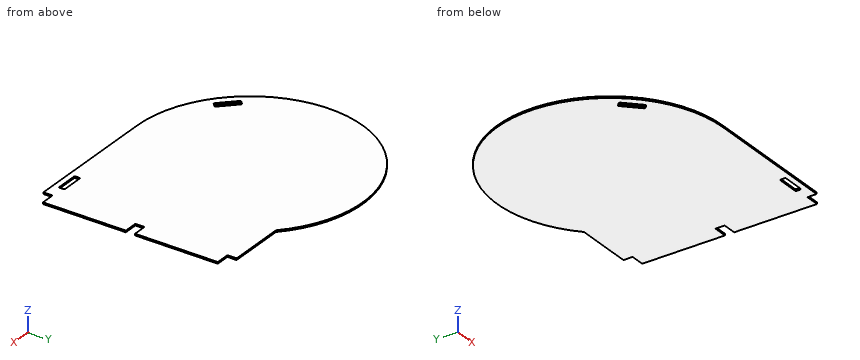
Autodesk Inventor part; units mm, degrees
ref_plane "YZ Plane" through (0, 0, 0) normal (1, 0, 0) x (0, 1, 0)
ref_plane "XZ Plane" through (0, 0, 0) normal (0, 1, 0) x (-1, 0, 0)
ref_plane "XY Plane" through (0, 0, 0) normal (0, 0, 1) x (1, 0, 0)
ref_plane "Work Plane1" through (0, 0, 0) normal (0, 0, 1) x (1, 0, 0)
sketch "Sketch1" plane through (0, 0, 0) normal (0, 0, 1) x (1, 0, 0)
  arc A0 (157.2336, 394.4305) -> (-185.695, -445.5695) centre (-185.695, 44.4305) ccw construction
  line L0 (404.305, 394.4305) -> (404.305, 354.4305) construction
  line L1 (404.305, 354.4305) -> (524.305, 354.4305) construction
  line L2 (524.305, -5.5695) -> (404.305, -5.5695) construction
  line L3 (404.305, -5.5695) -> (404.305, -45.5695) construction
  line L4 (404.305, -45.5695) -> (524.305, -45.5695) construction
  line L5 (404.305, -405.5695) -> (404.305, -445.5695) construction
  line L6 (524.305, -405.5695) -> (404.305, -405.5695) construction
  line L7 (-185.695, -445.5695) -> (464.305, -445.5695) construction
  line L8 (404.305, 394.4305) -> (404.305, 354.4305)
  line L9 (464.305, 354.4305) -> (404.305, 354.4305)
  line L10 (404.305, -5.5695) -> (464.305, -5.5695)
  line L11 (404.305, -5.5695) -> (404.305, -45.5695)
  line L12 (464.305, -45.5695) -> (404.305, -45.5695)
  line L13 (404.305, -405.5695) -> (464.305, -405.5695)
  line L14 (404.305, -405.5695) -> (404.305, -445.5695)
  line L15 (464.305, 354.4305) -> (464.305, -5.5695)
  line L16 (464.305, -45.5695) -> (464.305, -405.5695)
  line L17 (404.305, -445.5695) -> (-185.695, -445.5695)
  line L18 (157.2336, 394.4305) -> (404.305, 394.4305)
  arc A1 (157.2336, 394.4305) -> (-185.695, -445.5695) centre (-185.695, 44.4305) ccw
  arc A2 (-521.5707, -227.8057) -> (-528.6418, -227.8057) centre (-525.1062, -231.3412) ccw
  line L19 (-539.2484, -238.4123) -> (-528.6418, -227.8057)
  arc A3 (-539.2484, -238.4123) -> (-539.2484, -245.4833) centre (-535.7128, -241.9478) ccw
  line L20 (-475.6088, -309.1229) -> (-539.2484, -245.4833)
  line L21 (-521.5707, -227.8057) -> (-457.9311, -291.4453)
  arc A4 (-457.9311, -298.5163) -> (-457.9311, -291.4453) centre (-461.4666, -294.9808) ccw
  arc A5 (-475.6088, -309.1229) -> (-468.5377, -309.1229) centre (-472.0732, -305.5874) ccw
  line L22 (-457.9311, -298.5163) -> (-468.5377, -309.1229)
  line L23 (249.305, -395.5695) -> (339.305, -395.5695)
  arc A6 (344.305, -400.5695) -> (339.305, -395.5695) centre (339.305, -400.5695) ccw
  line L24 (344.305, -400.5695) -> (344.305, -415.5695)
  arc A7 (339.305, -420.5695) -> (344.305, -415.5695) centre (339.305, -415.5695) ccw
  line L25 (339.305, -420.5695) -> (249.305, -420.5695)
  arc A8 (244.305, -415.5695) -> (249.305, -420.5695) centre (249.305, -415.5695) ccw
  line L26 (244.305, -415.5695) -> (244.305, -400.5695)
  arc A9 (249.305, -395.5695) -> (244.305, -400.5695) centre (249.305, -400.5695) ccw
  point P0 (0, 0)
extrude "Extrusion1" add sketch "Sketch1" along normal blind 7
properties part number "Foam_Right"
Part model, mm, in its own coordinate system. Round coordinates to 2 decimals unless told otherwise and drop trailing zeros. Loops run counter-clockwise (first coordinate to the right, second up) from the corner with the lowest first, then second, coordinate; pieces in that order, holes last.
1. Flat gauge pins, fed straight in: pin 1 (2 mm diameter, centred on x = 292.5, z = 2.5, fed in from +Y); pin 2 (1.5 mm diameter, centred on x = -469.5, z = 4.5, fed in from -Y); pin 3 (3.5 mm diameter, centred on x = 447, z = 2.5, fed in from +Y). Where does each tip first touch, or does it go through?
Solutions:
pin 1: stops at y = 394.43
pin 2: stops at y = -355.54
pin 3: stops at y = 354.43
2. Drill centre lines: line 1 along Y through (x, z) = (272.5, 6.5); line 2 along X through (y, z) = (43, 5.25) (3 decimals); line 3 along Y through (x, z) = (365.5, 5.5). Where is each one in solid material? Low to high.
Solutions:
line 1: y = -445.57 to -420.57, -395.57 to 394.43
line 2: x = -675.693 to 464.305
line 3: y = -445.57 to 394.43
3. Slice it at B-B (y = -112). Give the cut face in (x, z) (3 decimals).
Solutions:
outline: (-650.054, 0) - (464.305, 0) - (464.305, 7) - (-650.054, 7) - close
4. Slice it at C-C (x = -424.5). Give the cut face in (y, z), and give its area (3 significant figures).
Solutions:
outline: (-383.44, 0) - (472.3, 0) - (472.3, 7) - (-383.44, 7) - close
area: 5,990 mm2
5. Slice it at A-A (z = 4). Give the cut face in (x, y) (1 decimal).
Solutions:
outline: (-185.7, -445.6) - (404.3, -445.6) - (404.3, -405.6) - (464.3, -405.6) - (464.3, -45.6) - (404.3, -45.6) - (404.3, -5.6) - (464.3, -5.6) - (464.3, 354.4) - (404.3, 354.4) - (404.3, 394.4) - (157.2, 394.4) arc R490 ccw (long way) to start; hole (-539.2, -245.5) - (-475.6, -309.1) arc R5 ccw to (-468.5, -309.1) - (-457.9, -298.5) arc R5 ccw to (-457.9, -291.4) - (-521.6, -227.8) arc R5 ccw to (-528.6, -227.8) - (-539.2, -238.4) arc R5 ccw to start; hole (244.3, -415.6) arc R5 ccw to (249.3, -420.6) - (339.3, -420.6) arc R5 ccw to (344.3, -415.6) - (344.3, -400.6) arc R5 ccw to (339.3, -395.6) - (249.3, -395.6) arc R5 ccw to (244.3, -400.6) - close
